Read the model definition and answer for the solid it produces. Units are mm, in the model's axes. Coordinates: 2 decimals unless noted, no trailing zeros. Write each loop counter-clockwise with the first axis right and the second up, starting at its lowest first coordinate (ties: lowest second). Pieces come first, ordered by that corner, then holes.
(1) Given pin 1 (10 mm diameter, centred on x = -43.5, z = 43, fed in from -Y); pin 2 (4 mm diameter, centred on y = 29, z = 79.5, fed in from -X); pin 3 (2 mm diameter, centred on x = -9, z = 26.5, fed in from -Y), each flat-ended and moving along its own axis, determine where each tip first touches the part or whether it passes through.
(2) Determine the mould class of faces 1 (the cylindrical face through (-60.47, -46.367, 53.219)), 2 (the flat face through (-1, 1, 0)) for opening direction X: pulls with the +X half, pulls with the -X half, needs draft (parallel to the pull), parting line crosses it, or undercut.
(3) The part is cut by section B-B, the plane x = -59.5. Determine the outline of the cut face in (y, z).
(4) Straight lines are drawn through the part: line 1 along Y through (x, z) = (15.5, 85); line 2 along Y through (x, z) = (-27.5, 11); line 3 along X through (y, z) = (-61, 61). For each, find the intervals that lie inside material, in ascending order.
(5) The part is cut by section C-C, the plane y = -60. Determine the outline of the cut face in (x, z), and give its area (3 significant figures).
(6) The part is cut by section A-A, the plane z = 80.5. Determine the outline of the cut face in (x, y), and give its area (3 significant figures).
```python
from build123d import *

# Parameters (mm, degrees)
F0_R     = 76.2
F1_DEPTH = 107.95
F2_R     = 15.820563
F3_DEPTH = 235.204
F4_R     = 29.432713
F5_DEPTH = 293.116


with BuildPart() as f1:
    # F0 (on Top) → F1 (new body)
    with BuildSketch(Plane.XY):
        Circle(F0_R)
    extrude(amount=F1_DEPTH)

    # F2 (on Top) → F3 (cut)
    with BuildSketch(Plane.XY):
        with Locations((-136.144727, 109.994054)):
            Circle(F2_R)
    extrude(amount=-F3_DEPTH, mode=Mode.SUBTRACT)

    # F4 (on Top) → F5 (cut)
    with BuildSketch(Plane.XY):
        Circle(F4_R)
    extrude(amount=-F5_DEPTH, mode=Mode.SUBTRACT)


solid = f1.part
```
Computed:
1. pin 1: stops at y = -65.76
1. pin 2: stops at x = -71.26
1. pin 3: stops at y = -75.78
2. face 1: parting line crosses it
2. face 2: needs draft
3. outline: (-47.6, 0) - (47.6, 0) - (47.6, 107.95) - (-47.6, 107.95) - close
4. line 1: y = -74.61 to 74.61
4. line 2: y = -71.06 to 71.06
4. line 3: x = -45.67 to 45.67
5. outline: (-46.97, 0) - (46.97, 0) - (46.97, 107.95) - (-46.97, 107.95) - close
5. area: 10,100 mm2
6. outline: circle Ø152.4 at (0, 0)
6. area: 18,200 mm2
